from build123d import *

# Parameters (mm, degrees)
SKETCH_1_W          = 20
SKETCH_1_H          = 3
EXTRUDE_1_DEPTH     = 660
SKETCH_2_R          = 1.575
CUT_EXTRUDE_1_DEPTH = 661.309775787


with BuildPart() as part:
    # 草图1 → 凸台-拉伸1 (new body)
    with BuildSketch(Plane.XY):
        with Locations((10, -1.5)):
            Rectangle(SKETCH_1_W, SKETCH_1_H)
    extrude(amount=EXTRUDE_1_DEPTH)

    # 草图2 → 切除-拉伸1 (cut, through all)
    with BuildSketch(Plane(origin=(0, 0, 0), x_dir=(1, 0, 0), z_dir=(0, 1, 0))):
        with Locations(Location((10, -10, 0), (0, 0, 270))):
            Circle(SKETCH_2_R)
        with Locations(Location((10, -30, 0), (0, 0, 270))):
            Circle(SKETCH_2_R)
        with Locations(Location((10, -50, 0), (0, 0, 270))):
            Circle(SKETCH_2_R)
        with Locations(Location((10, -70, 0), (0, 0, 270))):
            Circle(SKETCH_2_R)
        with Locations(Location((10, -90, 0), (0, 0, 270))):
            Circle(SKETCH_2_R)
        with Locations(Location((10, -110, 0), (0, 0, 270))):
            Circle(SKETCH_2_R)
        with Locations(Location((10, -130, 0), (0, 0, 270))):
            Circle(SKETCH_2_R)
        with Locations(Location((10, -150, 0), (0, 0, 270))):
            Circle(SKETCH_2_R)
        with Locations(Location((10, -170, 0), (0, 0, 270))):
            Circle(SKETCH_2_R)
        with Locations(Location((10, -190, 0), (0, 0, 270))):
            Circle(SKETCH_2_R)
        with Locations(Location((10, -210, 0), (0, 0, 270))):
            Circle(SKETCH_2_R)
        with Locations(Location((10, -230, 0), (0, 0, 270))):
            Circle(SKETCH_2_R)
        with Locations(Location((10, -250, 0), (0, 0, 270))):
            Circle(SKETCH_2_R)
        with Locations(Location((10, -270, 0), (0, 0, 270))):
            Circle(SKETCH_2_R)
        with Locations(Location((10, -290, 0), (0, 0, 270))):
            Circle(SKETCH_2_R)
        with Locations(Location((10, -310, 0), (0, 0, 270))):
            Circle(SKETCH_2_R)
        with Locations(Location((10, -330, 0), (0, 0, 270))):
            Circle(SKETCH_2_R)
        with Locations(Location((10, -350, 0), (0, 0, 270))):
            Circle(SKETCH_2_R)
        with Locations(Location((10, -370, 0), (0, 0, 270))):
            Circle(SKETCH_2_R)
        with Locations(Location((10, -390, 0), (0, 0, 270))):
            Circle(SKETCH_2_R)
        with Locations(Location((10, -410, 0), (0, 0, 270))):
            Circle(SKETCH_2_R)
        with Locations(Location((10, -430, 0), (0, 0, 270))):
            Circle(SKETCH_2_R)
        with Locations(Location((10, -450, 0), (0, 0, 270))):
            Circle(SKETCH_2_R)
        with Locations(Location((10, -470, 0), (0, 0, 270))):
            Circle(SKETCH_2_R)
        with Locations(Location((10, -490, 0), (0, 0, 270))):
            Circle(SKETCH_2_R)
        with Locations(Location((10, -510, 0), (0, 0, 270))):
            Circle(SKETCH_2_R)
        with Locations(Location((10, -530, 0), (0, 0, 270))):
            Circle(SKETCH_2_R)
        with Locations(Location((10, -550, 0), (0, 0, 270))):
            Circle(SKETCH_2_R)
        with Locations(Location((10, -570, 0), (0, 0, 270))):
            Circle(SKETCH_2_R)
        with Locations(Location((10, -590, 0), (0, 0, 270))):
            Circle(SKETCH_2_R)
        with Locations(Location((10, -610, 0), (0, 0, 270))):
            Circle(SKETCH_2_R)
        with Locations(Location((10, -630, 0), (0, 0, 270))):
            Circle(SKETCH_2_R)
        with Locations(Location((10, -650, 0), (0, 0, 270))):
            Circle(SKETCH_2_R)
    extrude(amount=-CUT_EXTRUDE_1_DEPTH, mode=Mode.SUBTRACT)


solid = part.part
Read the model definition and answer for the solid it produces. Units are mm, in the model's axes. Coordinates: 2 decimals unless noted, no trailing zeros. Answer in a Markdown table with one row per item.
Item 1: A cutting plane is placed at A-A on y = -0.7. Give the number of separate pieces and of enclosed holes in the cut face, plus the area to 3 significant figures.
Returned:
| item | result |
|---|---|
| separate pieces | 1 |
| enclosed holes | 33 |
| area | 12,900 mm^2 |
Item 2: Straight lines are drawn through the part: line 1 along X through (y, z) = (-1.45, 410) (3 decimals); line 2 along X through (y, z) = (-2.3, 610.5). For each, find the intervals that lie inside material, in ascending order. Write a range as [from, to].
Returned:
| item | result |
|---|---|
| line 1 | x = [0, 8.425], [11.575, 20] |
| line 2 | x = [0, 8.51], [11.49, 20] |
Item 3: This flat-tipped pin is pushed along its axis until it touches: P1, Ø5, axis at x = 9, z = 475.5, coming from the +Y side. Where does it stop, or does it pass through?
Returned:
| item | result |
|---|---|
| P1 | stops at y = 0 |
